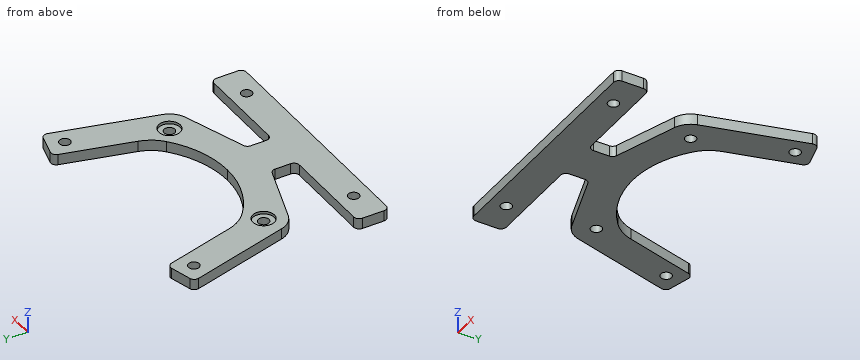
Autodesk Inventor part; units mm, degrees
ref_plane "YZ Plane" through (0, 0, 0) normal (1, 0, 0) x (0, 1, 0)
ref_plane "XZ Plane" through (0, 0, 0) normal (0, 1, 0) x (-1, 0, 0)
ref_plane "XY Plane" through (0, 0, 0) normal (0, 0, 1) x (1, 0, 0)
sketch "Sketch1" plane through (0, 0, 0) normal (0, 0, 1) x (1, 0, 0)
  circle A0 centre (-29, 0) radius 2
  line L0 (-62.2888, 0) -> (62.2888, 0) construction
  arc A1 (-36.7274, -2.0706) -> (-31.5768, -7.5737) centre (-29, 0) ccw
  arc A2 (-23.2301, 4.498) -> (0, -4) centre (0, 32) ccw
  line L1 (0, -55.9324) -> (0, 55.5944) construction
  line L2 (-31.5768, -7.5737) -> (-8.8558, -15.304)
  line L3 (-7.5, -17.1974) -> (-7.5, -23)
  line L4 (-36.7274, -2.0706) -> (-46.5625, 34.6346)
  line L5 (-45.1483, 37.0841) -> (-37.4209, 39.1547)
  line L6 (-34.9714, 37.7405) -> (-28.1342, 12.2236)
  arc A3 (-7.5, -17.1974) -> (-8.8558, -15.304) centre (-9.5, -17.1974) ccw
  arc A4 (-45.1483, 37.0841) -> (-46.5625, 34.6346) centre (-44.6307, 35.1523) ccw
  arc A5 (-34.9714, 37.7405) -> (-37.4209, 39.1547) centre (-36.9033, 37.2228) ccw
  circle A6 centre (29, 0) radius 2
  line L7 (62.2888, 0) -> (-62.2888, 0) construction
  arc A7 (31.5768, -7.5737) -> (36.7274, -2.0706) centre (29, 0) ccw
  line L8 (31.5768, -7.5737) -> (8.8558, -15.304)
  line L9 (7.5, -17.1974) -> (7.5, -25)
  line L10 (36.7274, -2.0706) -> (46.5625, 34.6346)
  line L11 (45.1483, 37.0841) -> (37.4209, 39.1547)
  arc A8 (8.8558, -15.304) -> (7.5, -17.1974) centre (9.5, -17.1974) ccw
  arc A9 (46.5625, 34.6346) -> (45.1483, 37.0841) centre (44.6307, 35.1523) ccw
  arc A10 (37.4209, 39.1547) -> (34.9714, 37.7405) centre (36.9033, 37.2228) ccw
  circle A11 centre (-29, 0) radius 4
  circle A12 centre (29, 0) radius 4
  line L12 (-9.5, -25) -> (-43, -25)
  line L13 (-45, -27) -> (-45, -35)
  line L14 (-43, -37) -> (0, -37)
  arc A13 (-43, -25) -> (-45, -27) centre (-43, -27) ccw
  arc A14 (-45, -35) -> (-43, -37) centre (-43, -35) ccw
  arc A15 (-9.5, -25) -> (-7.5, -23) centre (-9.5, -23) ccw
  line L15 (9.5, -25) -> (43, -25)
  line L16 (45, -27) -> (45, -35)
  line L17 (43, -37) -> (0, -37)
  arc A16 (45, -27) -> (43, -25) centre (43, -27) ccw
  arc A17 (43, -37) -> (45, -35) centre (43, -35) ccw
  arc A18 (7.5, -23) -> (9.5, -25) centre (9.5, -23) ccw
  arc A19 (-28.1342, 12.2236) -> (-23.2301, 4.498) centre (-13.3609, 16.1821) ccw
  arc A20 (0, -4) -> (23.2301, 4.498) centre (0, 32) ccw
  line L18 (34.9714, 37.7405) -> (28.1342, 12.2236)
  arc A21 (23.2301, 4.498) -> (28.1342, 12.2236) centre (13.3609, 16.1821) ccw
  circle A22 centre (-39.7317, 32.3238) radius 2
  circle A23 centre (39.7317, 32.3238) radius 2
  circle A24 centre (-33, -31) radius 2
  circle A25 centre (33, -31) radius 2
  point P0 (0, 0)
  point P1 (-7.5, -15.7653)
  point P2 (-47.0802, 36.5665)
  point P3 (-26.9294, 7.7274)
  point P4 (-7.5, -25)
  point P5 (-15, -20)
  point P6 (7.5, -15.7653)
  point P7 (47.0802, 36.5665)
  point P8 (15, -20)
  point P9 (-29, -40)
  point P10 (-45, -25)
  point P11 (-45, -37)
  point P12 (45, -25)
  point P13 (45, -37)
  point P14 (7.5, -23)
  dimension "d0" = 4
  dimension "d1" = 58
  dimension "d7" = 2
  dimension "d9" = 15
  dimension "d12" = 20
  dimension "d13" = 30
  dimension "d15" = 2
  dimension "d19" = 8
  dimension "d20" = 15
  dimension "d21" = 15
  dimension "d22" = 12
  dimension "d24" = 4
  dimension "d26" = 24
  dimension "d28" = 40
  dimension "d40" = 8
  dimension "d45" = 40
  dimension "d46" = 58
  dimension "d47" = 2
  dimension "d48" = 12
  dimension "d49" = 25
  dimension "d50" = 90
  dimension "d53" = 36
  dimension "d54" = 15.2944
  dimension "d55" = 4
  dimension "d56" = 6
  dimension "d57" = 6
  dimension "d61" = 4
  dimension "d62" = 12
  dimension "d63" = 6
extrude "Extrusion3" add sketch "Sketch1" along normal blind 3 contours A11 | A12
extrude "Extrusion4" add sketch "Sketch1" along normal blind 4 contours L4 A4 L5 A5 L6 A19 A2 A20 A21 L18 A10 L11 A9 L10 A7 L8 A8 L9 A18 L15 A16 L16 A17 L17 L14 A14 L13 A13 L12 A15 L3 A3 L2 A1
properties part number "UnitreeGO2_frontmount"
Input: part model. Units: mm. Frame: model coordinates. Round coordinates to 2 decimals unless told otherwise and drop trailing zeros. Loops run counter-clockwise (first coordinate to the right, second up) from the corner with the lowest first, then second, coordinate; pieces in that order, holes last. Notation, with made-up numbers: (57.5, -2) -> (79.5, -2) arc R33 cw to (79.5, 29) -> close; hole circle Ø3 at (-36, 14). An arc over 180 degrees is marked (long way). Write each question's results on one line, items separated by ' | '.
1. Ray query, line 1 (X direction, y = 2.5, z = 3.15); line 2 (X direction, y = -30, z = 1.7); line 3 (X direction, y = -17, z = 3.2). Return the intervals inside material, ascending. Write a range as from..to.
Geometry results:
line 1: -37.95..-32.12, -25.88..-20.63, 20.63..25.88, 32.12..37.95 | line 2: -45..-34.73, -31.27..31.27, 34.73..45 | line 3: -7.51..7.51
2. Section D-D (x = 12). Return loops of the section in (y, z).
Geometry results:
outline: (-37, 0) -> (-25, 0) -> (-25, 4) -> (-37, 4) -> close; (-14.23, 0) -> (-1.94, 0) -> (-1.94, 4) -> (-14.23, 4) -> close
3. Section B-B (x = -29.5). Return loops of the section in (y, z).
Geometry results:
outline: (-37, 0) -> (-25, 0) -> (-25, 4) -> (-37, 4) -> close; (-8.28, 0) -> (-1.94, 0) -> (-1.94, 3) -> (-3.97, 3) -> (-3.97, 4) -> (-8.28, 4) -> close; (1.94, 0) -> (17.32, 0) -> (17.32, 4) -> (3.97, 4) -> (3.97, 3) -> (1.94, 3) -> close
4. Section A-A (y = -31). Return loops of the section in (x, z), and give its area (3 significant figures).
Geometry results:
outline: (-45, 0) -> (-35, 0) -> (-35, 4) -> (-45, 4) -> close; (-31, 0) -> (31, 0) -> (31, 4) -> (-31, 4) -> close; (35, 0) -> (45, 0) -> (45, 4) -> (35, 4) -> close | area: 328 mm2
5. First-contact query: P1, Ø2.5, axis at x = -30, y = -1, coming from the +Z side; P2, Ø8, axis at x = 28.5, y = 31, coming from the +Z side; P3, Ø1.2, axis at x = -18, z = 2.5, coming from the +Y side; P4, Ø2, axis at y = -31.5, z = 2, coming from the -X side. Flat tips, straight axial feed; report the tip coordinate or a pass-through.
Geometry results:
P1: z = 3 | P2: through | P3: y = 1.18 | P4: x = -45
6. Section C-C (y = 17). Return loops of the section in (x, z).
Geometry results:
outline: (-41.84, 0) -> (-29.41, 0) -> (-29.41, 4) -> (-41.84, 4) -> close; (29.41, 0) -> (41.84, 0) -> (41.84, 4) -> (29.41, 4) -> close
